from build123d import *

# Parameters (mm, degrees)
SKETCH1_W           = 10
SKETCH1_H           = 10
BOSS_EXTRUDE1_DEPTH = 10
SKETCH1_3_W         = 10
SKETCH1_3_H         = 10
BOSS_EXTRUDE2_DEPTH = 5
SKETCH1_4_W         = 10
SKETCH1_4_H         = 10
BOSS_EXTRUDE3_DEPTH = 20
BOSS_EXTRUDE4_REACH = 85.066
SKETCH2_R           = 5
BOSS_EXTRUDE5_REACH = 76.833
SKETCH3_R           = 2.5


with BuildPart() as part:
    # Sketch1 → Boss-Extrude1 (new, symmetric)
    with BuildSketch(Plane.XY):
        Polygon((70, 0), (0, 0), (0, 40), (10, 40), (10, 20), (60, 20), (60, 40), (70, 40), align=None)
        with Locations((55, 10)):
            Rectangle(SKETCH1_W, SKETCH1_H, mode=Mode.SUBTRACT)
        with Locations((15, 10)):
            Rectangle(SKETCH1_W, SKETCH1_H, mode=Mode.SUBTRACT)
    extrude(amount=BOSS_EXTRUDE1_DEPTH, both=True)

    # Sketch1_3 → Boss-Extrude2 (add, symmetric)
    with BuildSketch(Plane.XY):
        with Locations((75, 10)):
            Rectangle(SKETCH1_3_W, SKETCH1_3_H)
        with Locations((-5, 10)):
            Rectangle(SKETCH1_3_W, SKETCH1_3_H)
    extrude(amount=BOSS_EXTRUDE2_DEPTH, both=True)

    # Sketch1_4 → Boss-Extrude3 (add, symmetric)
    with BuildSketch(Plane.XY):
        with Locations((15, 10)):
            Rectangle(SKETCH1_4_W, SKETCH1_4_H)
        with Locations((55, 10)):
            Rectangle(SKETCH1_4_W, SKETCH1_4_H)
    extrude(amount=BOSS_EXTRUDE3_DEPTH, both=True)

    # Sketch2 → Boss-Extrude4 (add, up to next)
    with BuildSketch(Plane(origin=(10, 0, 0), x_dir=(0, 0, -1), z_dir=(1, 0, 0)), mode=Mode.PRIVATE) as boss_extrude4_sk1:
        with Locations(Location((0, 30, 0), (0, 0, 180))):
            Circle(SKETCH2_R)
    boss_extrude4_tool1 = extrude(boss_extrude4_sk1.sketch, amount=BOSS_EXTRUDE4_REACH, mode=Mode.PRIVATE) - part.part
    add(boss_extrude4_tool1.solids().sort_by_distance((10, 30, 0))[0])

    # Sketch3 → Boss-Extrude5 (add, up to next)
    with BuildSketch(Plane(origin=(20, 0, 0), x_dir=(0, 0, -1), z_dir=(1, 0, 0)), mode=Mode.PRIVATE) as boss_extrude5_sk1:
        with Locations(Location((-15, 10, 0), (0, 0, 270))):
            Circle(SKETCH3_R)
    boss_extrude5_tool1 = extrude(boss_extrude5_sk1.sketch, amount=BOSS_EXTRUDE5_REACH, mode=Mode.PRIVATE) - part.part
    boss_extrude5 = boss_extrude5_tool1.solids().sort_by_distance((20, 10, 15))[0]
    add(boss_extrude5)

    # Mirror1: Boss-Extrude5 across plane
    add(boss_extrude5.mirror(Plane.XY))


solid = part.part
Check sheet for the modelled part. Datum: model origin and axes. Units: mm. A direction names the side the tool comes from. Give positions to 0.01 mm unless a question says otherwise; leave off trailing zeros. Order: outer loops, then holes, each group sorted by start corner. A loop starts at its lowest first (then second) coordinate and runs counter-clockwise, first axis right, second up. Notation, with made-up numbers: M 38,36 L 70,36 A20 cw 70,51 Z; hole C 64,42 d6. An arc over 180 degrees is marked long. Answer as CSV lines item,"result". Start each with the question number.
Item 1: Cross-section at A-A on x = 12. Enter the section's corners in (y, z).
Item 2: Tool access check on faces 1 (the face through (55, 5, -15)), 2 (the face through (-5, 10, 5)), 3 (the face through (10, 10, -15)), 4 (the face through (75, 10, -5)). Record the directions out of +Z, -Z, +X, -X, +Y, -Y that give a thin tool (end or side, any length) a straight path to the whole face; none if there is none.
Item 3: Thickness scan on line 1 (X direction, y = 34, z = 7.5); line 2 (X direction, y = 13, z = -15); line 3 (Z direction, x = 36, y = 6). Record the ranges inside material, lowest first. Write a range as [from, to].
Item 4: Cross-section at D-D on x = 24.5. Enter the section's corners in (y, z), plus the area to 3 significant figures.
Item 5: Gauge pin test, flat ends, axial feed: P1, Ø6, axis at y = 33, z = 1.5, coming from the -X side; P2, Ø1.5, axis at x = 32, y = 34.5, coming from the -Z side; P3, Ø5, axis at x = 58.5, z = 13.5, coming from the -Y side. Record the tip position at first contact, or that the pin passes through.
Item 6: Cross-section at C-C on z = -9. Enter the section's corners in (x, y), plus the area to 3 significant figures.
Item 7: Mould release check, pull along Y, two halves, no side actions. Record for faces 5 (the face through (55, 10, 20)), 6 (the face through (-5, 15, 0)), 7 (the face through (35, 20, 0)): +Y half, -Y half, draft (parallel to the pull), parting line (faces both ways), or undercut.
Item 8: Cross-section at B-B on y = 36.5. Enter the section's corners in (x, z), plus the area to 3 significant figures.
Established:
1,outline,"M 0,-10 L 5,-10 L 5,-20 L 15,-20 L 15,-10 L 20,-10 L 20,10 L 15,10 L 15,20 L 5,20 L 5,10 L 0,10 Z; C 30,0 d10"
2,face 1,"-Z, +X, -X, -Y"
2,face 2,"+Z, -X, +Y, -Y"
2,face 3,"-Z, -X, +Y, -Y"
2,face 4,"-Z, +X, +Y, -Y"
3,line 1,"x = [0, 10], [60, 70]"
3,line 2,"x = [10, 20], [50, 60]"
3,line 3,"z = [-10, 10]"
4,outline,"M 0,-10 L 20,-10 L 20,10 L 0,10 Z; C 10,-15 d5; C 10,15 d5; C 30,0 d10"
4,area,"518 mm^2"
5,P1,"stops at x = 0"
5,P2,"stops at z = -3.31"
5,P3,"stops at y = 5"
6,outline,"M 0,0 L 70,0 L 70,40 L 60,40 L 60,20 L 10,20 L 10,40 L 0,40 Z"
6,area,"1,800 mm^2"
7,face 5,"draft"
7,face 6,"+Y half"
7,face 7,"undercut"
8,outline,"M 0,-10 L 10,-10 L 10,10 L 0,10 Z; M 60,-10 L 70,-10 L 70,10 L 60,10 Z"
8,area,"400 mm^2"
